from build123d import *

# Parameters (mm, degrees)
IZIM1_W               = 120
IZIM1_H               = 12
IZIM2_W               = 120
IZIM2_H               = 8
KES_EKSTR_ZYON1_DEPTH = 18.3


with BuildPart() as part:
    # Çizim1 → Döndür1 (revolve)
    with BuildSketch(Plane.XY):
        with Locations((0, 21)):
            Rectangle(IZIM1_W, IZIM1_H)
    revolve(axis=Axis((-60, 0, 0), (1, 0, 0)))

    # Çizim2 → Kes-Ekstrüzyon1 (cut)
    with BuildSketch(Plane(origin=(0, 0, 0), x_dir=(1, 0, 0), z_dir=(0, 1, 0))):
        Rectangle(IZIM2_W, IZIM2_H)
    extrude(amount=-KES_EKSTR_ZYON1_DEPTH, mode=Mode.SUBTRACT)


solid = part.part
Design review of the part built by this model. Coordinates are the model's own, in mm. A direction names the side the tool comes from. Round coordinates to 2 decimals unless told otherwise and drop trailing zeros. Write each loop counter-clockwise with the first axis right and the second up, starting at its lowest first coordinate (ties: lowest second). Pieces come first, ordered by that corner, then holes.
Item 1: Wall thickness on L1, parallel to Z at x = 18, y = 0; L2, parallel to Y at x = 50.5, z = -6; L3, parallel to Y at x = -46, z = -9.5: over which ranges is each line inside the solid? List them lowest first.
Item 2: Consider section A-A on y = 0. Give the boundary of the cut face in (x, z).
Item 3: For faces 1 (the flat face through (-1, -18.3, 0)), 2 (the flat face through (60, -12, -12)), list the 3-axis set-ups (+Z, -Z, +X, -X, +Y, -Y) from which the entire face can be reached by the end or side of a thin tool; tool diameter is ignored.
Item 4: Consider section C-C on x = -31. Give the boundary of the cut face in (y, z), and give its area (3 significant figures).
Item 5: For pin 1 Ø1.2 at (x, y) = (-0.5, -16.5) entering from -Z; pin 2 Ø1.2 at (x, y) = (6, -16.5) entering from +Z; pin 3 Ø10 at (x, y) = (40, -2) entering from -Z, all flat-tipped, find the tip position at first contact; note any pin that passes through.
Item 6: Draft analysis for pull direction Y (two halves, no side actions). For faces 3 (the cylindrical face through (0.84, -5.85, -26.36)), 4 (the flat face through (-60, -12, -12)), 5 (the flat face through (-1, -16, 4)), state which applies: released by +Y, released by -Y, zero draft, split by the parting line, or undercut.
Item 7: Consider section B-B on z = 0. Give the boundary of the cut face in (x, y).
Check values:
1. L1: z = -27 to -15, 15 to 27
1. L2: y = -26.32 to -13.75, 13.75 to 26.32
1. L3: y = -25.27 to -11.61, 11.61 to 25.27
2. outline: (-60, -27) - (60, -27) - (60, -15) - (-60, -15) - close; (-60, 15) - (60, 15) - (60, 27) - (-60, 27) - close
3. face 1: +X, -X
3. face 2: +Z, -Z, +X, +Y, -Y
4. outline: circle Ø54 at (0, 0); hole (-18.3, -4) - (-14.46, -4) arc R15 ccw (long way) to (-14.46, 4) - (-18.3, 4) - close
4. area: 1,560 mm2
5. pin 1: stops at z = -21.82
5. pin 2: stops at z = 21.82
5. pin 3: stops at z = -27
6. face 3: split by the parting line
6. face 4: zero draft
6. face 5: undercut
7. outline: (-60, -27) - (60, -27) - (60, -18.3) - (-60, -18.3) - close; (-60, 15) - (60, 15) - (60, 27) - (-60, 27) - close
